Can you work these out from the drawing? Everything is in mm from the part's minimum corner. A direction names the side the tool comes from. Round coordinates to 2 decimals unless told otherwise and drop trailing zeros. Loops run counter-clockwise (first coordinate to the right, second up) from the corner with the lowest first, then second, coordinate; pieces in that order, holes last. Notation, with made-up numbers: M 74.5,73.5 L 81.5,73.5 A17 ccw 81.5,99.5 Z; hole C -17.75,-14.5 d3. An arc over 180 degrees is marked long. Answer in a Markdown table with one row per item.
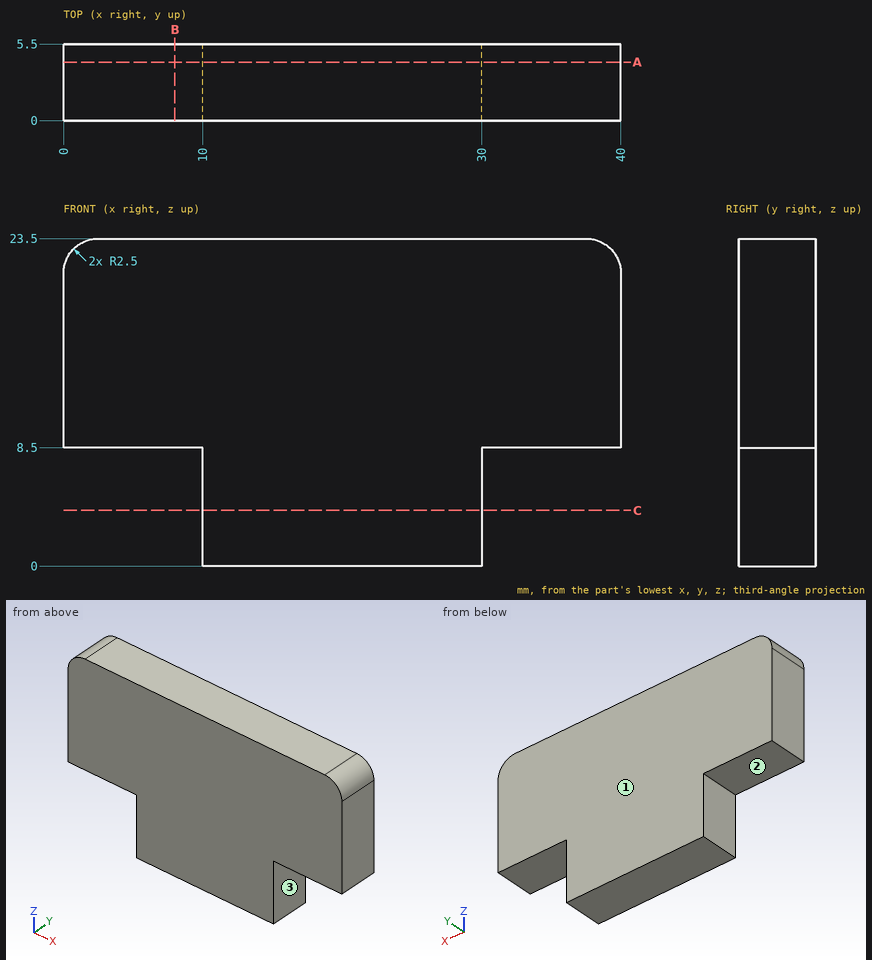
1) I want a section at A-A, the plane y = 4.2. Please give me the cut outline in (x, z), plus the area to 3 significant figures.
Computed:
| item | result |
|---|---|
| outline | M 0,8.5 L 10,8.5 L 10,0 L 30,0 L 30,8.5 L 40,8.5 L 40,21 A2.5 ccw 37.5,23.5 L 2.5,23.5 A2.5 ccw 0,21 Z |
| area | 767 mm² |
2) I want a section at C-C, the plane z = 4. Please give me the cut outline in (x, y), plus the area to 3 significant figures.
Computed:
| item | result |
|---|---|
| outline | M 10,0 L 30,0 L 30,5.5 L 10,5.5 Z |
| area | 110 mm² |
3) I want a section at B-B, the plane x = 8. Please give me the cut outline in (y, z).
Computed:
| item | result |
|---|---|
| outline | M 0,8.5 L 5.5,8.5 L 5.5,23.5 L 0,23.5 Z |
4) Will these pins go through, and if not, where does the flat tip stop? P1, Ø1.5, axis at y = 5, z = 6, coming from the -X side; P2, Ø3, axis at x = 33.5, y = 3.5, coming from the -Z side; P3, Ø3, axis at y = 3, z = 4, coming from the +X side.
Computed:
| item | result |
|---|---|
| P1 | stops at x = 10 |
| P2 | stops at z = 8.5 |
| P3 | stops at x = 30 |
5) Which directions (+Z, -Z, +X, -X, +Y, -Y) give clear straight access to the entire face, cutting with the end or side of a thin tool? Please do the marked faces 1, 2 and 3.
Computed:
| item | result |
|---|---|
| face 1 | +Z, -Z, +X, -X, +Y |
| face 2 | -Z, -X, +Y, -Y |
| face 3 | -Z, +X, +Y, -Y |
6) I need wall thicknesses on line 1 (X direction, y = 0.85, z = 2.75); line 2 (Z direction, x = 35, y = 0.65); line 3 (X direction, y = 4.6, z = 21.25). Which ranges of each line are inside material? Lowest first, please.
Computed:
| item | result |
|---|---|
| line 1 | x = 10 to 30 |
| line 2 | z = 8.5 to 23.5 |
| line 3 | x = 0.01 to 39.99 |
